Source: three-view drawing plus pictorial views. Frame: mm from the lowest corner of the part. Give positions to 0.01 mm unless a question says otherwise; leave off trailing zeros. Order: outer loops, then holes, each group sorted by start corner. A loop starts at its lowest first (then second) coordinate and runs counter-clockwise, first axis right, second up.
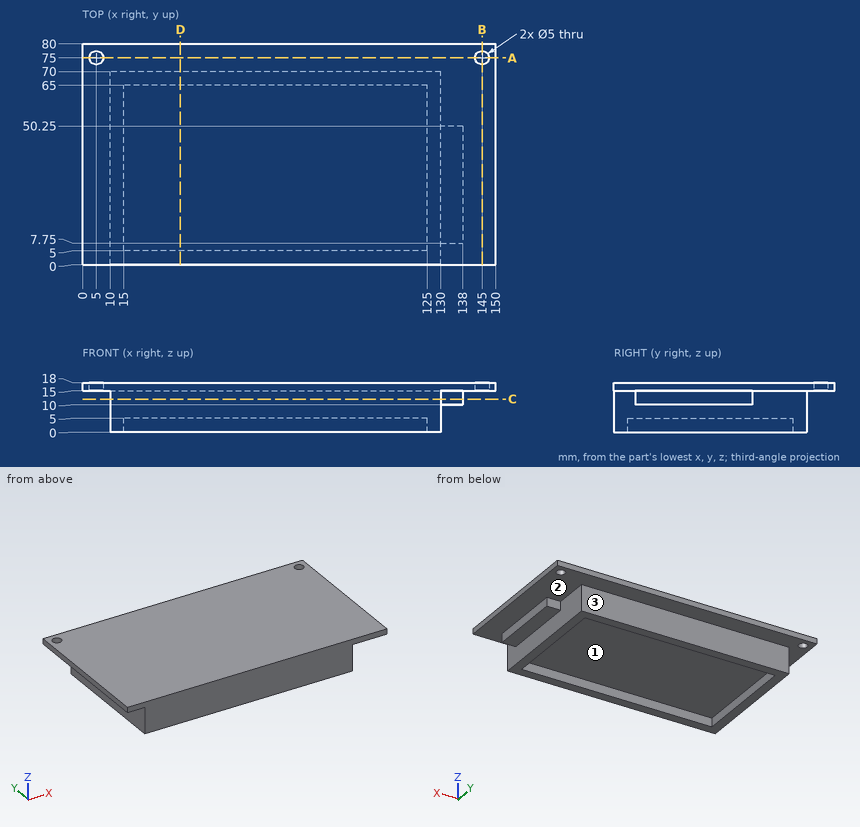
1) Section query C-C on z = 12. Output: boundary loops of the cut face in (x, y).
Checks:
outline: (10, 0) - (130, 0) - (130, 7.75) - (138, 7.75) - (138, 50.25) - (130, 50.25) - (130, 70) - (10, 70) - close
2) First-contact query: pin 1 Ø4 at (x, z) = (132.5, 13.5) entering from -Y; pin 2 Ø1 at (y, z) = (10.5, 6) entering from +X; pin 3 Ø2.5 at (x, z) = (132.5, 12) entering from +Y; pin 4 Ø5.5 at (y, z) = (23.5, 2) entering from -X. Flat tips, straight axial feed; report the tip coordinate or a pass-through.
Checks:
pin 1: stops at y = 0
pin 2: stops at x = 130
pin 3: stops at y = 50.25
pin 4: stops at x = 10
3) Section query D-D on x = 35.5. Output: boundary loops of the cut face in (y, z), and give its area (3 significant figures).
Checks:
outline: (0, 0) - (5, 0) - (5, 5) - (65, 5) - (65, 0) - (70, 0) - (70, 15) - (80, 15) - (80, 18) - (0, 18) - close
area: 990 mm2
4) Section query A-A on y = 75. Output: boundary loops of the cut face in (x, z).
Checks:
outline: (0, 15) - (2.5, 15) - (2.5, 18) - (0, 18) - close; (7.5, 15) - (142.5, 15) - (142.5, 18) - (7.5, 18) - close; (147.5, 15) - (150, 15) - (150, 18) - (147.5, 18) - close
5) Pull-direction query (Y, two-part tool) for the marked faces 1, 2 and 3; classes: +Y half, -Y half, draft (parallel to the pull), parting line (faces both ways), or undercut.
Checks:
face 1: undercut
face 2: draft
face 3: +Y half
6) Ray query, L1, parallel to X at y = 26.5, z = 4.5; L2, parallel to Y at x = 5, z = 15.85; L3, parallel to Y at x = 22, z = 5.5. Return the intervals inside material, ascending.
Checks:
L1: x = 10 to 15, 125 to 130
L2: y = 0 to 72.5, 77.5 to 80
L3: y = 0 to 70
7) Section query B-B on x = 145. Output: boundary loops of the cut face in (y, z).
Checks:
outline: (0, 15) - (72.5, 15) - (72.5, 18) - (0, 18) - close; (77.5, 15) - (80, 15) - (80, 18) - (77.5, 18) - close
